Read the model definition and answer for the solid it produces. Units are mm, in the model's axes. Face numbers are marked on the shaded views. A direction names the side the tool comes from. Give positions to 0.01 mm unless a question says otherwise; leave off trailing zeros. Loops run counter-clockwise (first coordinate to the right, second up) from the corner with the lowest first, then second, coordinate; pieces in that order, holes last. Notation, with made-up numbers: (-28, -19.5) - (12, -19.5) arc R27 ccw to (12, 4.5) - close; hole circle Ø9 at (4.25, 22). An arc over 180 degrees is marked (long way). Write item = value, one per line.
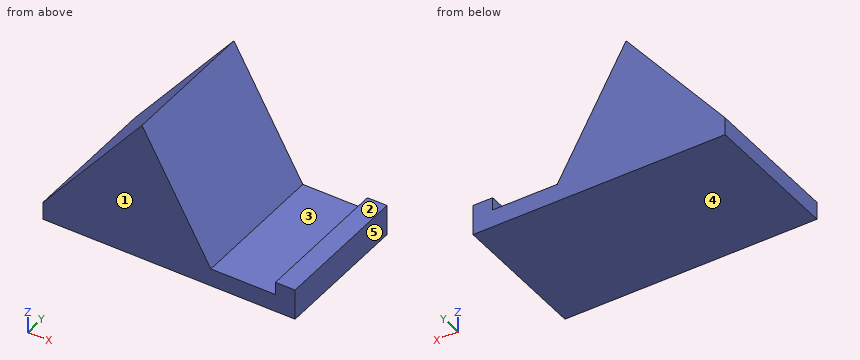
```python
from build123d import *

# Parameters (mm, degrees)
F0_W     = 3.5603952128
F0_H     = 2.3265234751
F1_DEPTH = 25.4


with BuildPart() as f1:
    # F0 (on Front) → F1 (new body)
    with BuildSketch(Plane.XZ):
        Polygon((-45.72, 0), (0, 0), (0, 3.2118688712), (-3.5603952128, 3.2118688712), (-15.2750396183, 3.2118688712), (-45.72, 3.2118688712), align=None)
        with Locations((-1.7801976064, 4.3751306088)):
            Rectangle(F0_W, F0_H)
        Polygon((-27.766545563, 25.327977915), (-45.72, 3.2118688712), (-15.2750396183, 3.2118688712), align=None)
    extrude(amount=F1_DEPTH)


solid = f1.part
```
1) A cutting plane is placed at C-C on z = 15. Determine the outline of the cut face in (x, y).
Output:
outline = (-36.15, -25.4) - (-21.93, -25.4) - (-21.93, 0) - (-36.15, 0) - close
2) Find the intervals of material crossed by probe 1 along Z at (x, y) = (-6, -10.75); probe 2 along X at (y, z) = (-14, 5) (3 decimals); probe 3 along X at (y, z) = (-18.5, 22.5), in increasing order.
Output:
probe_1 = 0 to 3.21
probe_2 = -44.268 to -16.285, -3.56 to 0
probe_3 = -30.06 to -26.17
3) A cutting plane is placed at A-A on y = -22.5. Determine the outline of the cut face in (x, z), then the cut area to 3 significant figures.
Output:
outline = (-45.72, 0) - (0, 0) - (0, 5.54) - (-3.56, 5.54) - (-3.56, 3.21) - (-15.28, 3.21) - (-27.77, 25.33) - (-45.72, 3.21) - close
area = 492 mm²
4) A cutting plane is placed at B-B on x = -36. Determine the outline of the cut face in (y, z).
Output:
outline = (-25.4, 0) - (0, 0) - (0, 15.19) - (-25.4, 15.19) - close
5) Each of these flat-tipped pins is pushed along its axis until it touches: P1, Ø4, axis at x = -2, y = -16.5, coming from the +Z side; P2, Ø4, axis at y = -17.5, z = 11, coming from the +X side; P3, Ø10, axis at x = -19, y = -3.5, coming from the +Z side; P4, Ø2, axis at x = -17.5, z = 11, coming from the +Y side. Where does it stop, or does it pass through?
Output:
P1 = 5.54
P2 = -18.54
P3 = 18.66
P4 = through
6) The mould has two halves that part along X. Classify the marked faces 3, 4 and 5: pulls with the +X half, pulls with the -X half, needs draft (parallel to the pull), parting line crosses it, or undercut.
Output:
face_3 = undercut
face_4 = needs draft
face_5 = pulls with the +X half
7) A tool of negligible diameter and unlimited length cuts with its end or side. For the marked faces 1 and 2, from which of +Z, -Z, +X, -X, +Y, -Y can it reach the whole face along a straight path? Write none if from no direction.
Output:
face_1 = +Z, -Z, +X, -X, -Y
face_2 = +Z, +X, +Y, -Y
